Here's how the part is built. I have some questions about the finished solid (model axes, mm). A direction names the side the tool comes from. Coordinates: 2 decimals unless noted, no trailing zeros. Order: outer loops, then holes, each group sorted by start corner. A loop starts at its lowest first (then second) coordinate and runs counter-clockwise, first axis right, second up. Notation, with made-up numbers: (-38.5, 13) -> (7.5, 13) arc R10 ccw to (7.5, 21) -> close; hole circle Ø2 at (56.5, 43). An arc over 180 degrees is marked (long way). One line per item, written item: value. Start each with the question number.
```python
from build123d import *

# Parameters (mm, degrees)
SKETCH001_W   = 112
SKETCH001_H   = 44
PAD_DEPTH     = 2
SKETCH_R      = 2
SKETCH_R_2    = 0.825
PAD001_DEPTH  = 6.5
SKETCH002_W   = 112
SKETCH002_H   = 44
SKETCH002_W_2 = 108
SKETCH002_H_2 = 40
PAD002_DEPTH  = 25
POCKET_DEPTH  = 5
FILLET_R      = 2


with BuildPart() as part:
    # Sketch001 → Pad (new body)
    with BuildSketch(Plane.XY):
        Rectangle(SKETCH001_W, SKETCH001_H)
    extrude(amount=PAD_DEPTH)

    # Sketch → Pad001 (join)
    with BuildSketch(Plane.XY):
        with Locations((51.201135, 16.51)):
            Circle(SKETCH_R)
        with Locations((51.201135, 16.51)):
            Circle(SKETCH_R_2, mode=Mode.SUBTRACT)
        with Locations((5.481135, 16.51)):
            Circle(SKETCH_R)
        with Locations((5.481135, 16.51)):
            Circle(SKETCH_R_2, mode=Mode.SUBTRACT)
        with Locations((-4.518865, 16.51)):
            Circle(SKETCH_R)
        with Locations((-4.518865, 16.51)):
            Circle(SKETCH_R_2, mode=Mode.SUBTRACT)
        with Locations((-51.018865, 16.51)):
            Circle(SKETCH_R)
        with Locations((-51.018865, 16.51)):
            Circle(SKETCH_R_2, mode=Mode.SUBTRACT)
        with Locations((-51.018865, -16.51)):
            Circle(SKETCH_R)
        with Locations((-51.018865, -16.51)):
            Circle(SKETCH_R_2, mode=Mode.SUBTRACT)
        with Locations((-4.518865, -16.51)):
            Circle(SKETCH_R)
        with Locations((-4.518865, -16.51)):
            Circle(SKETCH_R_2, mode=Mode.SUBTRACT)
        with Locations((5.481135, -16.51)):
            Circle(SKETCH_R)
        with Locations((5.481135, -16.51)):
            Circle(SKETCH_R_2, mode=Mode.SUBTRACT)
        with Locations((51.201135, -16.51)):
            Circle(SKETCH_R)
        with Locations((51.201135, -16.51)):
            Circle(SKETCH_R_2, mode=Mode.SUBTRACT)
    extrude(amount=PAD001_DEPTH)

    # Sketch002 (on Face5 of Pad001) → Pad002 (join)
    with BuildSketch(Plane.XY.offset(2)):
        Rectangle(SKETCH002_W, SKETCH002_H)
        Rectangle(SKETCH002_W_2, SKETCH002_H_2, mode=Mode.SUBTRACT)
    extrude(amount=PAD002_DEPTH)

    # Sketch003 (on Face8 of Pad002) → Pocket (cut)
    with BuildSketch(Plane.YZ.offset(56)):
        with BuildLine():
            ThreePointArc((-5.554717, 25), (-13.101596, 17.453121), (-5.554717, 9.906242))
            Line((-5.554717, 9.906242), (5.554717, 9.906242))
            ThreePointArc((5.554717, 9.906242), (13.101596, 17.453121), (5.554717, 25))
            Line((5.554717, 25), (-5.554717, 25))
        make_face()
    extrude(amount=-POCKET_DEPTH, mode=Mode.SUBTRACT)

    # Fillet
    fillet_edges = [part.edges().sort_by_distance(p)[0] for p in [
        (56, -22, 14.5),
        (56, 22, 14.5),
        (-56, -22, 14.5),
        (-56, 22, 14.5),
    ]]
    fillet(fillet_edges, radius=FILLET_R)


solid = part.part
```
Q1. Imagine slicing it at A-A (y = -3). Write out the boundary of the cut face in (x, z), plus the area to 3 significant figures.
Q2. If we mould it in two halves opening along Z, with no side actions, what happens to faces 1 (the face through (55, -13.1, 17.6)), 2 (the face through (56, 0, 7)), 3 (the face through (52.1, 16.1, 6.5))? For each: +Z half, -Z half, draft (parallel to the pull), parting line (faces both ways), or undercut.
Q3. I need wall thicknesses on line 1 (Y direction, x = -49, z = 20); line 2 (Y direction, x = -3.5, z = 4); line 3 (X direction, y = -12, z = 25.75). Which ranges of each line are inside material? Lowest first, please.
Q4. For faces 4 (the face through (55, 13.1, 17.3)), 5 (the face through (-50, -16, 6.5)), 6 (the face through (-56, 0, 13)), which set-ups out of +Z, -Z, +X, -X, +Y, -Y let a thin tool reach every point of the face, with its end or its side?
Q5. Imagine slicing it at D-D (y = 11.5). Write out the boundary of the cut face in (x, z), plus the area to 3 significant figures.
Q6. Imagine slicing it at C-C (z = 16.5). Write out the boundary of the cut face in (x, y).
Q7. For P1, Ø4.5, axis at x = -5, y = 16.5, coming from the +Z side; P2, Ø1.5, axis at y = 1.5, z = 21.5, coming from the +X side; P3, Ø3, axis at x = -14, y = -13, coming from the +Z side, each with a flat end and sliding along its axis, tell me the tip position at first contact or that it passes through.
Q8. Imagine slicing it at B-B (x = -46). Write out the boundary of the cut face in (y, z).
Completed:
1. outline: (-56, 0) -> (56, 0) -> (56, 9.91) -> (54, 9.91) -> (54, 2) -> (-54, 2) -> (-54, 27) -> (-56, 27) -> close; (54, 25) -> (56, 25) -> (56, 27) -> (54, 27) -> close
1. area: 294 mm2
2. face 1: undercut
2. face 2: draft
2. face 3: +Z half
3. line 1: y = -22 to -20, 20 to 22
3. line 2: y = -22 to -20, -18.23 to -14.79, 14.79 to 18.23, 20 to 22
3. line 3: x = -56 to -54, 54 to 56
4. face 4: +X
4. face 5: +Z
4. face 6: +Z, -Z, -X, +Y, -Y
5. outline: (-56, 0) -> (56, 0) -> (56, 12.8) -> (54, 12.8) -> (54, 2) -> (-54, 2) -> (-54, 27) -> (-56, 27) -> close; (54, 22.1) -> (56, 22.1) -> (56, 27) -> (54, 27) -> close
5. area: 305 mm2
6. outline: (-56, -20) arc R2 ccw to (-54, -22) -> (54, -22) arc R2 ccw to (56, -20) -> (56, -13.04) -> (54, -13.04) -> (54, -20) -> (-54, -20) -> (-54, 20) -> (54, 20) -> (54, 13.04) -> (56, 13.04) -> (56, 20) arc R2 ccw to (54, 22) -> (-54, 22) arc R2 ccw to (-56, 20) -> close
7. P1: stops at z = 6.5
7. P2: stops at x = -54
7. P3: stops at z = 2
8. outline: (-22, 0) -> (22, 0) -> (22, 27) -> (20, 27) -> (20, 2) -> (-20, 2) -> (-20, 27) -> (-22, 27) -> close
